Here's the drawing with two shaded views (mm, measured from the low corner). I have some questions. Give positions to 0.01 mm unless a question says otherwise; leave off trailing zeros. Loops run counter-clockwise (first coordinate to the right, second up) from the corner with the lowest first, then second, coordinate; pieces in that order, holes last. Notation, with made-up numbers: M 72.5,-26.5 L 94.5,-26.5 A38 ccw 94.5,11.5 Z; hole C -23.75,26.5 d6. An arc over 180 degrees is marked long. Put each result on its own line as item: value. Start each with the question number.
1) Imagine slicing it at C-C (z = 1.05). Write out the boundary of the cut face in (x, y) (3 decimals), then the cut area to 3 significant figures.
2) Imagine slicing it at B-B (x = 18.5). Write out the boundary of the cut face in (y, z), then the cut area to 3 significant figures.
3) Imagine slicing it at D-D (x = 26). Write out the boundary of the cut face in (y, z).
4) Please list where these lines run through material, in increasing order: line 1 along Y through (x, z) = (25, 1.65); line 2 along X through (y, z) = (16, 0.95); line 3 along Y through (x, z) = (42, 0.8). Write a range as from..to.
5) For P1, Ø3, axis at x = 8.76, y = 15.62, coming from the +Z side; P2, Ø1, axis at x = 22, z = 2, coming from the -Y side, each with a flat end and sliding along its axis, tell me the tip position at first contact or that it passes through.
6) Imagine slicing it at A-A (y = 25). Write out the boundary of the cut face in (x, z), then the cut area to 3 significant figures.
7) If we mould it in two halves opening along X, with no side actions, what happens to the marked faces 1, 2 and 3? For each: +X half, -X half, draft (parallel to the pull), parting line (faces both ways), or undercut.
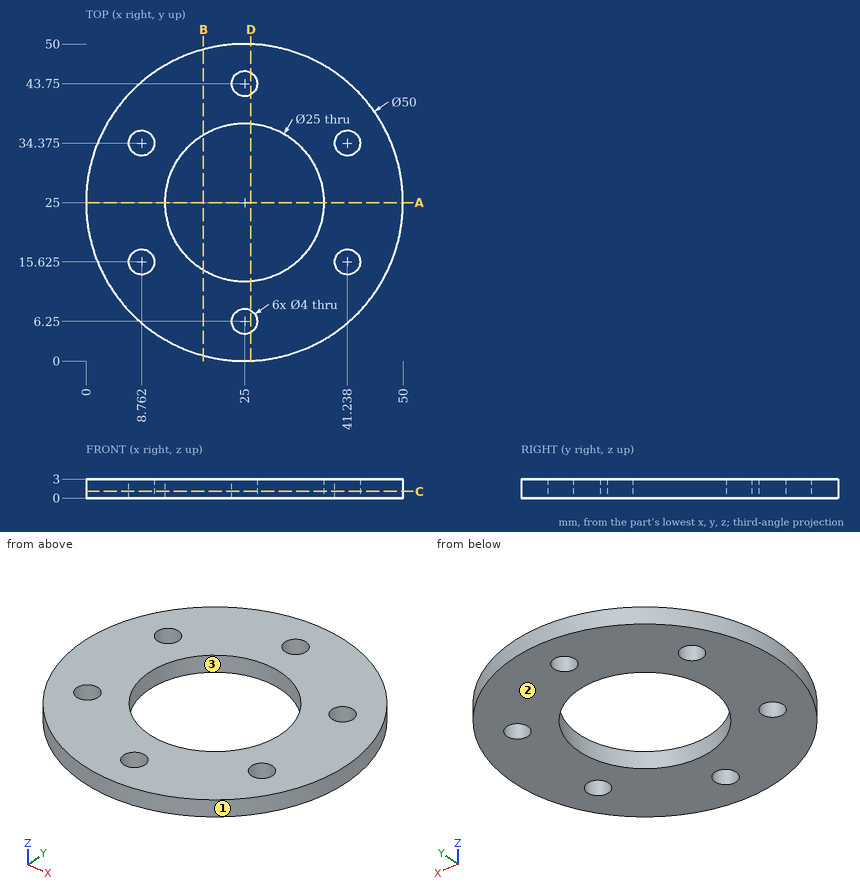
Recorded:
1. outline: C 25,25 d50; hole C 8.762,15.625 d4; hole C 8.762,34.375 d4; hole C 25,25 d25; hole C 25,6.25 d4; hole C 25,43.75 d4; hole C 41.238,15.625 d4; hole C 41.238,34.375 d4
1. area: 1,400 mm²
2. outline: M 0.86,0 L 14.32,0 L 14.32,3 L 0.86,3 Z; M 35.68,0 L 49.14,0 L 49.14,3 L 35.68,3 Z
2. area: 80.8 mm²
3. outline: M 0.02,0 L 4.52,0 L 4.52,3 L 0.02,3 Z; M 7.98,0 L 12.54,0 L 12.54,3 L 7.98,3 Z; M 37.46,0 L 42.02,0 L 42.02,3 L 37.46,3 Z; M 45.48,0 L 49.98,0 L 49.98,3 L 45.48,3 Z
4. line 1: 0..4.25, 8.25..12.5, 37.5..41.75, 45.75..50
4. line 2: 1.68..6.8, 10.73..16.33, 33.67..39.27, 43.2..48.32
4. line 3: 6.67..13.78, 17.47..32.53, 36.22..43.33
5. P1: through
5. P2: y = 0.13
6. outline: M 0,0 L 12.5,0 L 12.5,3 L 0,3 Z; M 37.5,0 L 50,0 L 50,3 L 37.5,3 Z
6. area: 75.0 mm²
7. face 1: parting line
7. face 2: draft
7. face 3: undercut
